Build history of the part. All positions in model axes, mm. Coordinates: 2 decimals unless noted, no trailing zeros. Order: outer loops, then holes, each group sorted by start corner. A loop starts at its lowest first (then second) coordinate and runs counter-clockwise, first axis right, second up. Notation, with made-up numbers: (48.25, 3) - (90.25, 3) arc R17 cw to (90.25, 14) - close; hole circle Ø8 at (12.5, 84.25). An arc over 180 degrees is marked (long way). Return JSON: item names as keys, results as strings.
from build123d import *

# Parameters (mm, degrees)
SKETCH1_W = 3
SKETCH1_H = 1.2065
SKETCH2_R = 0.127


with BuildPart() as part:
    # Sketch1 → Revolve1 (revolve)
    with BuildSketch(Plane.XY):
        with Locations((-1.5, 0.60325)):
            Rectangle(SKETCH1_W, SKETCH1_H)
    revolve(axis=Axis((0, 0, 0), (1, 0, 0)))

    # Sweep1: sweep along a path in Sketch3
    with BuildLine(Plane(origin=(0, 0, 0), x_dir=(1, 0, 0), z_dir=(0, 1, 0))) as sweep1_path:
        Line((0, 0), (2, 0))
        ThreePointArc((2, 0), (3.414213562, -0.585786438), (4, -2))
        Line((4, -2), (4, -78.2))
    # Sketch2 → Sweep1 (sweep)
    with BuildSketch(Plane(origin=(0, 0, 0), x_dir=(0, 0, -1), z_dir=(1, 0, 0))):
        with Locations((0, 1.0795)):
            Circle(SKETCH2_R)
        with Locations((0, -1.0795)):
            Circle(SKETCH2_R)
    sweep(path=sweep1_path.line)


solid = part.part
1. Cut at B-B on y = 0. Give the cut face in (x, z).
Check values:
{"outline": "(-3, -1.21) - (0, -1.21) - (0, 1.21) - (-3, 1.21) - close"}
2. Probe L1, parallel to Y at x = 4, z = 53.5; L2, parallel to Z at x = -1.5, y = 0.55; L3, parallel to Z at x = -1, y = -0.3. List the from-to ranges inside material, lowest first.
Check values:
{"L1": "-1.21 to -0.95, 0.95 to 1.21", "L2": "-1.07 to 1.07", "L3": "-1.17 to 1.17"}
3. Cut at C-C on x = 1.25. Give the cut face in (y, z), plus the area to 3 significant figures.
Check values:
{"outline": "circle Ø0.25 at (-1.08, 0); circle Ø0.25 at (1.08, 0)", "area": "0.101 mm²"}
4. Cut at D-D on x = -2.25. Give the cut face in (y, z).
Check values:
{"outline": "circle Ø2.41 at (0, 0)"}
5. Cut at A-A on z = 38.5. Give the cut face in (x, y).
Check values:
{"outline": "circle Ø0.25 at (4, -1.08); circle Ø0.25 at (4, 1.08)"}
